from build123d import *

# Parameters (mm, degrees)
SKETCH1_W           = 38.1
SKETCH1_H           = 19.05
SKETCH1_W_2         = 31.75
SKETCH1_H_2         = 12.7
BOSS_EXTRUDE1_DEPTH = 304.8
SKETCH2_R           = 14.2875
CUT_EXTRUDE1_DEPTH  = 20.05
SKETCH3_R           = 3.175
CUT_EXTRUDE2_DEPTH  = 20.05
CUT_EXTRUDE3_DEPTH  = 20.05
SKETCH5_R           = 2.667
CUT_EXTRUDE4_DEPTH  = 20.05
CUT_EXTRUDE5_REACH  = 21.05
SKETCH6_R           = 6.35


with BuildPart() as part:
    # Sketch1 → Boss-Extrude1 (new body)
    with BuildSketch(Plane.XY):
        with Locations((19.05, 9.525)):
            Rectangle(SKETCH1_W, SKETCH1_H)
        with Locations((19.05, 9.525)):
            Rectangle(SKETCH1_W_2, SKETCH1_H_2, mode=Mode.SUBTRACT)
    extrude(amount=BOSS_EXTRUDE1_DEPTH)

    # Sketch2 → Cut-Extrude1 (cut, through all)
    with BuildSketch(Plane(origin=(0, 19.05, 0), x_dir=(1, 0, 0), z_dir=(0, 1, 0))):
        with Locations((19.05, -19.05)):
            Circle(SKETCH2_R)
        with Locations((19.05, -222.25)):
            Circle(SKETCH2_R)
    extrude(amount=-CUT_EXTRUDE1_DEPTH, mode=Mode.SUBTRACT)

    # Sketch3 → Cut-Extrude2 (cut, through all)
    with BuildSketch(Plane(origin=(0, 19.05, 0), x_dir=(1, 0, 0), z_dir=(0, 1, 0))):
        with Locations((19.05, -295.275)):
            Circle(SKETCH3_R)
    extrude(amount=-CUT_EXTRUDE2_DEPTH, mode=Mode.SUBTRACT)

    # Sketch4 → Cut-Extrude3 (cut, through all)
    with BuildSketch(Plane(origin=(0, 19.05, 0), x_dir=(1, 0, 0), z_dir=(0, 1, 0))):
        with BuildLine():
            Line((30.774464213, -304.8), (30.774464213, -247.65))
            ThreePointArc((30.774464213, -247.65), (32.920063969, -242.470063969), (38.1, -240.324464213))
            Line((38.1, -240.324464213), (38.1, -304.8))
            Line((38.1, -304.8), (30.774464213, -304.8))
        make_face()
    extrude(amount=-CUT_EXTRUDE3_DEPTH, mode=Mode.SUBTRACT)

    # Sketch5 → Cut-Extrude4 (cut, through all)
    with BuildSketch(Plane(origin=(0, 19.05, 0), x_dir=(1, 0, 0), z_dir=(0, 1, 0))):
        with Locations((19.05, -120.65)):
            Circle(SKETCH5_R)
    extrude(amount=-CUT_EXTRUDE4_DEPTH, mode=Mode.SUBTRACT)

    # Sketch6 → Cut-Extrude5 (cut, up to next)
    with BuildSketch(Plane.XZ, mode=Mode.PRIVATE) as cut_extrude5_sk1:
        with Locations((19.05, 120.65)):
            Circle(SKETCH6_R)
    cut_extrude5_tool1 = extrude(cut_extrude5_sk1.sketch, amount=-CUT_EXTRUDE5_REACH, mode=Mode.PRIVATE) & part.part
    add(cut_extrude5_tool1.solids().sort_by_distance((19.05, 0, 120.65))[0], mode=Mode.SUBTRACT)


solid = part.part
Can you work these out from the model? Positions are in its coordinate system, mm. A direction names the side the tool comes from. Give positions to 0.01 mm unless a question says otherwise; leave off trailing zeros. Loops run counter-clockwise (first coordinate to the right, second up) from the corner with the lowest first, then second, coordinate; pieces in that order, holes last. Notation, with made-up numbers: M 66,-21.75 L 87,-21.75 A27 ccw 87,-1.75 Z; hole C 56,-12 d9. An arc over 180 degrees is marked long. One line per item, written item: value. Start each with the question number.
1) On a 3-axis mill with a long thin cutter (end or side, diameter ignored), from which of +Z, -Z, +X, -X, +Y, -Y can I reach the whole of each face in a straight line? I mean faces 4 (the face through (22.464, 1.565, 126.004)), 5 (the face through (36.126, 9.658, 240.595)), 6 (the face through (3.175, 9, 150)). Say none if no direction works.
2) I'm going to push flat-ended pins straight in: pin 1 (2.5 mm diameter, centred on y = 1.5, z = 270.5, fed in from +X); pin 2 (5 mm diameter, centred on x = 19.05, z = 295.275, fed in from -Y); pin 3 (6 mm diameter, centred on x = 19.05, z = 120.65, fed in from -Y) (3 decimals). Where does each tip first touch, or does it pass through?
3) If I drill on line 1 (Z direction, x = 19.05, y = 16.5); line 2 (Y direction, x = 24.5, z = 51.5) (3 decimals); line 3 (X direction, y = 2.05, z = 222.25), over which ranges is the centre line in solid material (lowest first)? Write a range as [from, to].
4) If we section it at C-C, the plane y = 7.5: Write out the boundary of the cut face in (x, z) (3 decimals), and give its area (3 significant figures).
5) Thinking about a two-plate mould opening in X: for faces 1 (the face through (38.1, 9, 118)), 2 (the face through (32.68, 1.61, 14.76)), 3 (the face through (19, 0, 150)), which applies, +X half, -X half, draft (parallel to the pull), parting line (faces both ways), or undercut?
6) If we section it at A-A, the plane z = 196: Write out the boundary of the cut face in (x, y) (3 decimals).
7) If we section it at B-B, the plane z = 120.65: Write out the boundary of the cut face in (x, y) (3 decimals), and give its area (3 significant figures).
8) If we section it at D-D, the plane z = 259.5: Write out the boundary of the cut face in (x, y) (3 decimals), and give its area (3 significant figures).
Completed:
1. face 4: -Y
1. face 5: +Z, +X, +Y, -Y
1. face 6: +Z, -Z
2. pin 1: stops at x = 30.77
2. pin 2: passes through
2. pin 3: stops at y = 15.875
3. line 1: z = [0, 4.76], [33.34, 117.98], [123.32, 207.96], [236.54, 292.1], [298.45, 304.8]
3. line 2: y = [0, 3.175], [15.875, 19.05]
3. line 3: x = [0, 4.76], [33.34, 38.1]
4. outline: M 0,0 L 3.175,0 L 3.175,304.8 L 0,304.8 Z; M 34.925,0 L 38.1,0 L 38.1,240.324 A7.326 cw 34.925,241.048 Z
4. area: 1,730 mm^2
5. face 1: +X half
5. face 2: undercut
5. face 3: draft
6. outline: M 0,0 L 38.1,0 L 38.1,19.05 L 0,19.05 Z; hole M 3.175,3.175 L 34.925,3.175 L 34.925,15.875 L 3.175,15.875 Z
7. outline: M 0,0 L 12.7,0 L 12.7,3.175 L 3.175,3.175 L 3.175,15.875 L 16.383,15.875 L 16.383,19.05 L 0,19.05 Z; M 21.717,15.875 L 34.925,15.875 L 34.925,3.175 L 25.4,3.175 L 25.4,0 L 38.1,0 L 38.1,19.05 L 21.717,19.05 Z
7. area: 265 mm^2
8. outline: M 0,0 L 30.774,0 L 30.774,3.175 L 3.175,3.175 L 3.175,15.875 L 30.774,15.875 L 30.774,19.05 L 0,19.05 Z
8. area: 236 mm^2
